The listing builds one solid part. Answer for the finished solid, in the listing's coordinates (mm). A direction names the side the tool comes from. Round coordinates to 2 decimals unless told otherwise and drop trailing zeros. Loops run counter-clockwise (first coordinate to the right, second up) from the corner with the lowest first, then second, coordinate; pieces in that order, holes last. Notation, with made-up numbers: (-34, 40.25) - (16, 40.25) arc R28 ccw to (16, 60.25) - close; hole circle Ø5 at (19, 38.5). An arc over 180 degrees is marked (long way). One line per item, written item: value.
```python
from build123d import *

# Parameters (mm, degrees)
SKETCH1_W           = 100
SKETCH1_H           = 100
BOSS_EXTRUDE1_DEPTH = 4
SKETCH9_W           = 100
SKETCH9_H           = 100
BOSS_EXTRUDE2_DEPTH = 4
SKETCH10_W          = 100
SKETCH10_H          = 100
BOSS_EXTRUDE3_DEPTH = 4


with BuildPart() as part:
    # Sketch1 → Boss-Extrude1 (new body)
    with BuildSketch(Plane.XY.offset(50)):
        Rectangle(SKETCH1_W, SKETCH1_H)
        Polygon((-43.171572875, 46), (43.171572875, 46), (0, 2.828427125), align=None, mode=Mode.SUBTRACT)
        Polygon((46, -43.171572875), (46, 43.171572875), (2.828427125, 0), align=None, mode=Mode.SUBTRACT)
        Polygon((-43.171572875, -46), (43.171572875, -46), (0, -2.828427125), align=None, mode=Mode.SUBTRACT)
        Polygon((-46, -43.171572875), (-46, 43.171572875), (-2.828427125, 0), align=None, mode=Mode.SUBTRACT)
    extrude(amount=-BOSS_EXTRUDE1_DEPTH)


with BuildPart() as body_2:
    # Mirror2: mirrored copy
    add(part.part.mirror(Plane.XY))


with BuildPart() as part_1:
    add(part.part)

    add(body_2.part)  # Boss-Extrude2 merges body 2
    # Sketch9 → Boss-Extrude2 (add)
    with BuildSketch(Plane(origin=(50, 0, 0), x_dir=(0, 0, -1), z_dir=(1, 0, 0))):
        Rectangle(SKETCH9_W, SKETCH9_H)
        Polygon((43.171572875, 46), (-43.171572875, 46), (0, 2.828427125), align=None, mode=Mode.SUBTRACT)
        Polygon((-46, -43.171572875), (-46, 43.171572875), (-2.828427125, 0), align=None, mode=Mode.SUBTRACT)
        Polygon((43.171572875, -46), (-43.171572875, -46), (0, -2.828427125), align=None, mode=Mode.SUBTRACT)
        Polygon((46, -43.171572875), (46, 43.171572875), (2.828427125, 0), align=None, mode=Mode.SUBTRACT)
    boss_extrude2 = extrude(amount=-BOSS_EXTRUDE2_DEPTH)

    # Mirror3: Boss-Extrude2 across plane
    add(boss_extrude2.mirror(Plane(origin=(0, 0, 0), x_dir=(0, 0, 1), z_dir=(1, 0, 0))))

    # Sketch10 → Boss-Extrude3 (add)
    with BuildSketch(Plane(origin=(0, 50, 0), x_dir=(1, 0, 0), z_dir=(0, 1, 0))):
        Rectangle(SKETCH10_W, SKETCH10_H)
        Polygon((-46, -43.171572875), (-46, 43.171572875), (-2.828427125, 0), align=None, mode=Mode.SUBTRACT)
        Polygon((-43.171572875, 46), (43.171572875, 46), (0, 2.828427125), align=None, mode=Mode.SUBTRACT)
        Polygon((46, -43.171572875), (46, 43.171572875), (2.828427125, 0), align=None, mode=Mode.SUBTRACT)
        Polygon((-43.171572875, -46), (43.171572875, -46), (0, -2.828427125), align=None, mode=Mode.SUBTRACT)
    extrude(amount=BOSS_EXTRUDE3_DEPTH)


solid = part_1.part
```
1) A cutting plane is placed at B-B on x = -17. Give the number of separate pieces and of enclosed holes in the cut face, and give its area (3 significant figures).
Final values:
separate pieces: 10
enclosed holes: 0
area: 232 mm2
2) For a pull along Z with two mould halves and no side action, classify faces 4 (the flat face through (21.89, -24.72, 48.03)), 5 (the flat face through (-21.28, 51.97, 24.11)), 6 (the flat face through (-24.11, 51.97, 21.28)) as released by +Z, released by -Z, zero draft, split by the parting line, or undercut.
Final values:
face 4: zero draft
face 5: undercut
face 6: undercut
3) Consider L1, parallel to Z at x = 31, y = 48; L2, parallel to Y at x = -21, z = 20. Determine where each line is inside the solid, lowest interval first.
Final values:
L1: -50 to -46, 46 to 50
L2: 50 to 54
4) A cutting plane is placed at A-A on y = 48.5. Give the vertices of the cut face in (x, z).
Final values:
outline: (-50, -50) - (50, -50) - (50, 50) - (-50, 50) - close; hole (-46, -46) - (46, -46) - (46, 46) - (-46, 46) - close
5) Each of these flat-tipped pins is pushed along its axis until it touches: pin 1 Ø12 at (x, y) = (26, -8) entering from -Z; pin 2 Ø3 at (x, z) = (-15.5, -15.5) entering from -Y; pin 3 Ø12 at (x, z) = (34.5, 31) entering from +Y. Where does it stop, or does it pass through?
Final values:
pin 1: through
pin 2: y = 50
pin 3: y = 54
6) For faces 1 (the flat face through (-24.11, -21.28, 48.03)), 2 (the flat face through (-21.28, 51.97, -24.11)), 3 (the flat face through (48, 1, -46)), determine the directions among +Z, -Z, +X, -X, +Y, -Y from which every point of the face is accessible in a straight line to the end or side of a thin tool.
Final values:
face 1: +Z, -Z
face 2: +Y, -Y
face 3: +X, -X
